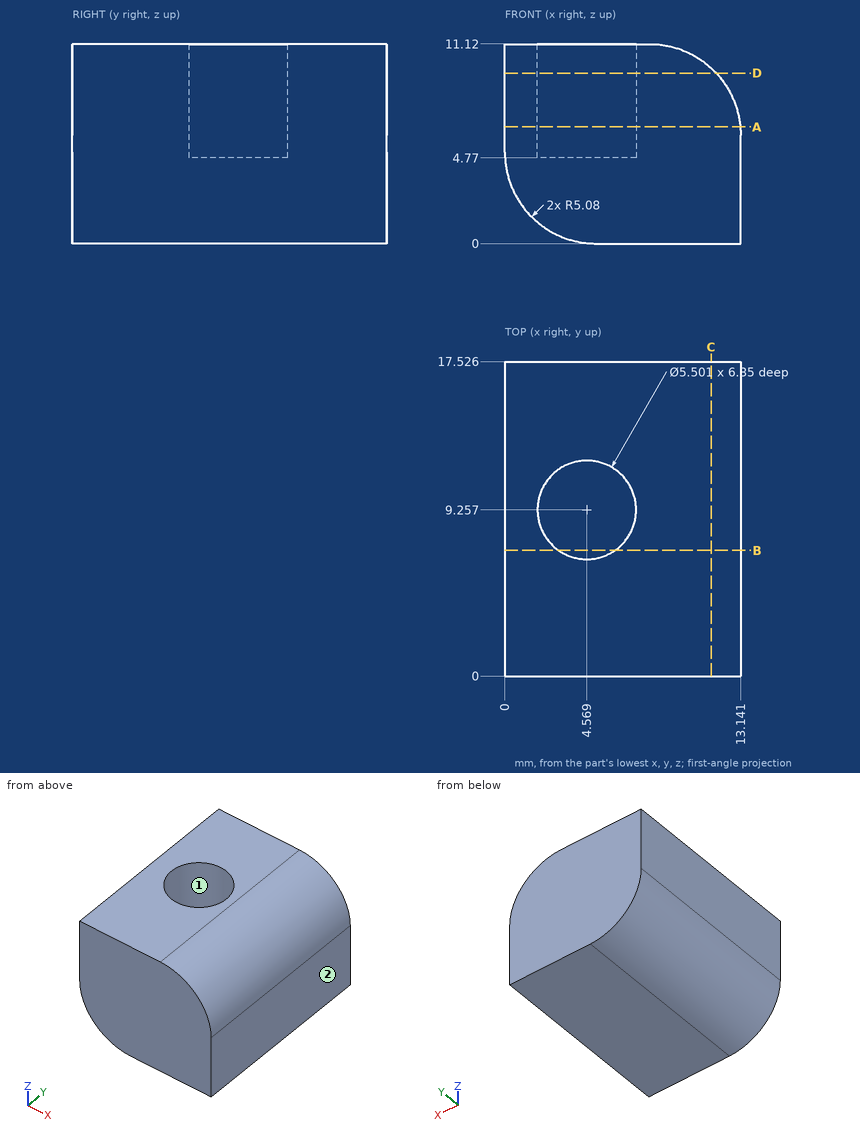
Input: dimensioned drawing with shaded views. Units: mm. Origin: part minimum x, y, z. A direction names the side the tool comes from. Coordinates: 2 decimals unless noted, no trailing zeros. Loops run counter-clockwise (first coordinate to the right, second up) from the corner with the lowest first, then second, coordinate; pieces in that order, holes last. Notation, with made-up numbers: (39, 18) -> (80, 18) arc R30 ccw to (80, 45) -> close; hole circle Ø1 at (44.5, -13.75). An arc over 180 degrees is marked (long way). One line per item, written item: value. Start each with the question number.
Q1. Section query A-A, the plane z = 6.5. Return the cut outline in (x, y).
Q2. Line query: line 1 along Y through (x, z) = (4.5, 10.75); line 2 along Y through (x, z) = (3.25, 6.25) (1 decimal); line 3 along X through (y, z) = (13.5, 6.25). Output: solid intervals per line, ascending.
Q3. Set-up query: the marked faces 1 and 2. Return all of +Z, -Z, +X, -X, +Y, -Y with unobstructed straight access to the full face (end or side cutting, diameter ignored); none if empty.
Q4. Section query B-B, the plane y = 7. Return the cut outline in (x, z).
Q5. Section query C-C, the plane x = 11.5. Return the cut outline in (y, z).
Q6. Section query D-D, the plane z = 9.5. Return the cut outline in (x, y).
Results:
1. outline: (0, 0) -> (13.12, 0) -> (13.12, 17.53) -> (0, 17.53) -> close; hole circle Ø5.5 at (4.57, 9.26)
2. line 1: 0 to 6.51, 12.01 to 17.53
2. line 2: 0 to 6.8, 11.7 to 17.5
2. line 3: 0 to 13.14
3. face 1: +Z
3. face 2: +Z, -Z, +X, +Y, -Y
4. outline: (0, 5.08) arc R5.08 ccw to (5.08, 0) -> (13.14, 0) -> (13.14, 6.04) arc R5.08 ccw to (8.06, 11.12) -> (6.14, 11.12) -> (6.14, 4.77) -> (3, 4.77) -> (3, 11.12) -> (0, 11.12) -> close
5. outline: (0, 0) -> (17.53, 0) -> (17.53, 9.78) -> (0, 9.78) -> close
6. outline: (0, 0) -> (11.78, 0) -> (11.78, 17.53) -> (0, 17.53) -> close; hole circle Ø5.5 at (4.57, 9.26)
